Design review of the part built by this model. Coordinates are the model's own, in mm. A direction names the side the tool comes from. Round coordinates to 2 decimals unless told otherwise and drop trailing zeros. Loops run counter-clockwise (first coordinate to the right, second up) from the corner with the lowest first, then second, coordinate; pieces in that order, holes last. Notation, with made-up numbers: (77, 25.25) - (133, 25.25) arc R22 cw to (133, 54.25) - close; hole circle Ø1 at (36, 42). An arc over 180 degrees is marked (long way). Return JSON: item names as keys, results as strings. Group by question number.
Autodesk Inventor part; units mm, degrees
ref_plane "YZ Plane" through (0, 0, 0) normal (1, 0, 0) x (0, 1, 0)
ref_plane "XZ Plane" through (0, 0, 0) normal (0, 1, 0) x (-1, 0, 0)
ref_plane "XY Plane" through (0, 0, 0) normal (0, 0, 1) x (1, 0, 0)
sketch "Skizze1" plane through (0, 0, 0) normal (0, 0, 1) x (1, 0, 0)
  line L0 (-24, 0) -> (144, 0)
  line L1 (0, -32) -> (0, 192)
  line L2 (0, 0) -> (120, 0)
  line L3 (120, 0) -> (120, 160)
  line L4 (120, 160) -> (0, 160)
  line L5 (0, 160) -> (0, 0)
  point P0 (0, 160)
  dimension "d0" = 120
  dimension "d1" = 160
extrude "Extrusion1" add sketch "Skizze1" along normal blind 285
sketch "Skizze2" plane through (0, 160, 0) normal (0, 1, 0) x (1, 0, 0)
  point P0 (0, 0)
sketch "Skizze3" plane through (0, 0, 285) normal (0, 0, 1) x (1, 0, 0)
  line L0 (10, 40) -> (110, 40)
  line L1 (110, 40) -> (110, 10)
  line L2 (110, 10) -> (10, 10)
  line L3 (10, 10) -> (10, 40)
  line L4 (0, 0) -> (120, 0)
  line L5 (120, 0) -> (120, 160)
  line L6 (0, 160) -> (0, 0)
  dimension "d4" = 10
  dimension "d5" = 10
  dimension "d6" = 10
  dimension "d7" = 30
extrude "Extrusion2" cut sketch "Skizze3" against normal blind 275
sketch "Skizze4" plane through (0, 160, 0) normal (0, 1, 0) x (1, 0, 0)
  point P0 (0, 0)
sketch "Skizze5" plane through (0, 160, 0) normal (0, 1, 0) x (1, 0, 0)
  line L0 (10, -10) -> (110, -10)
  line L1 (110, -10) -> (110, -275)
  line L2 (110, -275) -> (10, -275)
  line L3 (10, -275) -> (10, -10)
  line L4 (10, -190) -> (110, -190)
  line L5 (120, 0) -> (0, 0)
  line L6 (10, -100) -> (110, -100)
  line L7 (10, -185) -> (110, -185)
  line L8 (120, -285) -> (0, -285)
  line L9 (10, -95) -> (110, -95)
  line L10 (0, 0) -> (0, -285)
  line L11 (120, 0) -> (120, -285)
  dimension "d10" = 10
  dimension "d11" = 10
  dimension "d12" = 5
  dimension "d13" = 85
  dimension "d14" = 85
  dimension "d15" = 5
  dimension "d16" = 85
  dimension "d17" = 10
  dimension "d18" = 10
extrude "Extrusion3" cut sketch "Skizze5" against normal blind 110 contours L0 L1 L9 L3 | L6 L1 L7 L3 | L4 L1 L2 L3
sketch "Skizze6" plane through (0, 160, 0) normal (0, 1, 0) x (1, 0, 0)
  line L0 (7.5, -7.5) -> (112.5, -7.5)
  line L1 (112.5, -7.5) -> (112.5, -277.5)
  line L2 (112.5, -277.5) -> (7.5, -277.5)
  line L3 (7.5, -277.5) -> (7.5, -7.5)
  line L4 (2.5, -2.5) -> (117.5, -2.5)
  line L5 (117.5, -2.5) -> (117.5, -282.5)
  line L6 (117.5, -282.5) -> (2.5, -282.5)
  line L7 (2.5, -282.5) -> (2.5, -2.5)
  line L8 (120, 0) -> (120, -285)
  line L9 (110, -190) -> (110, -275)
  line L10 (110, -275) -> (10, -275)
  line L11 (120, -285) -> (0, -285)
  line L12 (10, -275) -> (10, -190)
  line L13 (0, 0) -> (0, -285)
  line L14 (120, 0) -> (0, 0)
  line L15 (10, -10) -> (110, -10)
  dimension "d21" = 2.5
  dimension "d22" = 2.5
  dimension "d23" = 2.5
  dimension "d24" = 2.5
  dimension "d25" = 2.5
  dimension "d26" = 2.5
  dimension "d27" = 2.5
  dimension "d28" = 2.5
extrude "Extrusion4" cut sketch "Skizze6" against normal blind 5 contours L4 L5 L6 L7
properties part number "EierkocherTeil1" material "Acetalharz, Schwarz"
Q1. Draft analysis for pull direction Z (two halves, no side actions). For faces 4 (the flat face through (10, 106, 233)), 5 (the flat face through (59, 99, 285)), 6 (the flat face through (10, 25, 149)), state which applies: pulls with the +Z half, pulls with the -Z half, needs draft (parallel to the pull), parting line crosses it, or undercut.
Q2. Add section B-B, the plane y = 81. State the section outline as (x, z) points.
Q3. Insertion check: pin 1 Ø1.5 at (x, y) = (40.5, 21.5) entering from +Z; pin 2 Ø2 at (x, z) = (101, 166) entering from +Y. Each pin has a flat end and moves straight along its axis. Give the tip position at first contact, or say it passes through.
Q4. Add section A-A, the plane z = 34.5. State the section outline as (x, y) points.
Q5. For line 1 (Z direction, x = 94.5, y = 54.5); line 2 (X direction, y = 108.5, z = 58.5); line 3 (Y direction, x = 90, z = 134), list the stretches that pass through material, from the lowest coordinate up.
Q6. Add section C-C, the plane x = 21. State the section outline as (y, z) points, plus the area to 3 significant figures.
Q7. Tool access review of faces 1 (the flat face through (110, 25, 149)), 2 (the flat face through (9.7, 160, 141.9)), 3 (the flat face through (59, 106, 95)): name each direction out of +Z, -Z, +X, -X, +Y, -Y from which nothing blocks a thin tool from reaching the whole face with its end or side.
Evaluation:
{
 "1": {"face 4": "undercut", "face 5": "pulls with the +Z half", "face 6": "needs draft"},
 "2": {"outline": "(0, 0) - (120, 0) - (120, 285) - (0, 285) - close; hole (10, 10) - (110, 10) - (110, 95) - (10, 95) - close; hole (10, 100) - (110, 100) - (110, 185) - (10, 185) - close; hole (10, 190) - (110, 190) - (110, 275) - (10, 275) - close"},
 "3": {"pin 1": "z = 10", "pin 2": "y = 50"},
 "4": {"outline": "(0, 0) - (120, 0) - (120, 160) - (117.5, 160) - (117.5, 155) - (112.5, 155) - (112.5, 160) - (110, 160) - (110, 50) - (10, 50) - (10, 160) - (7.5, 160) - (7.5, 155) - (2.5, 155) - (2.5, 160) - (0, 160) - close; hole (10, 10) - (110, 10) - (110, 40) - (10, 40) - close"},
 "5": {"line 1": "0 to 10, 95 to 100, 185 to 190, 275 to 285", "line 2": "0 to 10, 110 to 120", "line 3": "0 to 10, 40 to 50"},
 "6": {"outline": "(0, 0) - (160, 0) - (160, 2.5) - (155, 2.5) - (155, 7.5) - (160, 7.5) - (160, 10) - (50, 10) - (50, 95) - (160, 95) - (160, 100) - (50, 100) - (50, 185) - (160, 185) - (160, 190) - (50, 190) - (50, 275) - (160, 275) - (160, 277.5) - (155, 277.5) - (155, 282.5) - (160, 282.5) - (160, 285) - (40, 285) - (40, 10) - (10, 10) - (10, 285) - (0, 285) - close", "area": "9,250 mm²"},
 "7": {"face 1": "+Z", "face 2": "+Z, -Z, +X, -X, +Y", "face 3": "+Y"}
}
